Autodesk Inventor part; units mm, degrees
ref_plane "Work Plane1" through (0, 1.5, 0) normal (0, -1, 0) x (1, 0, 0)
ref_plane "YZ Plane" through (0, 0, 0) normal (1, 0, 0) x (0, 1, 0)
ref_plane "XZ Plane" through (0, 0, 0) normal (0, 1, 0) x (-1, 0, 0)
sketch "Sketch1" plane through (0, 0, 0) normal (0, 1, 0) x (-1, 0, 0)
  line L0 (0, 0) -> (29.5, 0)
  line L1 (29.5, 0) -> (29.5, -36.2)
  line L2 (29.5, -36.2) -> (0, -36.2)
  line L3 (0, -36.2) -> (0, 0)
  dimension "d0" = 29.5
  dimension "d1" = 36.2
extrude "Extrusion1" add sketch "Sketch1" along normal blind 5
sketch "Sketch2" plane through (0, 5, 0) normal (0, 1, 0) x (1, 0, 0)
  line L0 (-29.5, 0) -> (0, 0)
  line L1 (-14.75, 0) -> (-14.75, 17.5)
  arc A0 (-18.4298, 18.4481) -> (-11.0702, 18.4481) centre (-14.75, 17.5) ccw
  line L2 (-14.75, 17.5) -> (-14.75, 23.5)
  arc A1 (-11.0702, 18.4481) -> (-18.4298, 18.4481) centre (-14.75, 23.5) ccw
  circle A2 centre (-14.75, 23.5) radius 12.175
  circle A3 centre (-14.75, 23.5) radius 14.75
  dimension "d4" = 17.5
  dimension "d5" = 7.6
  dimension "d6" = 6
  dimension "d7" = 12.5
  dimension "d8" = 24.35
  dimension "d9" = 29.5
extrude "Extrusion2" add sketch "Sketch2" along normal blind 3.8 contours A2 | A3
sketch "Sketch4" plane through (-14.75, 8.8, -23.5) normal (0, 1, 0) x (1, 0, 0)
  circle A0 centre (0, 0) radius 12.25
  circle A1 centre (0, 0) radius 14.7438
  point P0 (14.75, -23.5)
  dimension "d12" = 24.5
extrude "Extrusion3" add sketch "Sketch4" along normal blind 6
sketch "Sketch5" plane through (-14.75, 8.8, -23.5) normal (0, 1, 0) x (1, 0, 0)
  arc A0 (-3.6798, -5.0519) -> (3.6798, -5.0519) centre (0, -6) ccw
  arc A1 (3.6798, -5.0519) -> (-3.6798, -5.0519) centre (0, 0) ccw
  point P0 (14.75, -23.5)
extrude "Extrusion4" cut sketch "Sketch5" against normal up to surface (8.8 mm away)
sketch "Sketch6" plane through (0, 0, 0) normal (0, -1, 0) x (1, 0, 0)
  arc A0 (-11.0702, -18.4481) -> (-18.4298, -18.4481) centre (-14.75, -17.5) ccw
  arc A1 (-18.4298, -18.4481) -> (-11.0702, -18.4481) centre (-14.75, -23.5) ccw
  line L0 (0, 0) -> (-29.5, 0)
  line L1 (-29.5, 0) -> (-29.5, -36.2)
  line L2 (-29.5, -36.2) -> (0, -36.2)
  line L3 (0, -36.2) -> (0, 0)
  line L4 (-14.75, 0) -> (-14.75, -36.2)
  line L5 (0, -36.2) -> (0, 0)
  line L6 (0, -18.1) -> (-29.5, -18.1)
  line L7 (-21.0275, -1.55) -> (-8.4725, -1.55)
  line L8 (-8.4725, -1.55) -> (-8.4725, -34.65)
  line L9 (-8.4725, -34.65) -> (-21.0275, -34.65)
  line L10 (-21.0275, -34.65) -> (-21.0275, -1.55)
  line L11 (-21.0275, -1.55) -> (-8.4725, -34.65) construction
  line L12 (-8.4725, -1.55) -> (-21.0275, -34.65) construction
  point P0 (-14.75, -18.1)
  dimension "d17" = 12.555
  dimension "d18" = 33.1
extrude "Extrusion5" cut sketch "Sketch6" against normal blind 6 contours A0 L6 L8 L9 L4 A1 | A0 L4 L7 L8 L6 | L4 L9 L10 L6 A0 A1 | A0 L6 L10 L7 L4
ref_plane "Work Plane1" through (0, 1.5, 0) normal (0, -1, 0) x (1, 0, 0)
sketch "Sketch7" plane through (0, 1.5, 0) normal (0, -1, 0) x (1, 0, 0)
  line L0 (-8.4725, -1.55) -> (-8.4725, -34.65)
  line L1 (-8.4725, -34.65) -> (-21.0275, -34.65)
  line L2 (-21.0275, -1.55) -> (-8.4725, -1.55)
  line L3 (-21.0275, -34.65) -> (-21.0275, -1.55)
  line L4 (-8.4725, -1.55) -> (-21.0275, -1.55)
  line L5 (-21.0275, -1.55) -> (-21.0275, -6.091)
  line L6 (-21.0275, -6.091) -> (-8.4725, -6.091)
  line L7 (-8.4725, -6.091) -> (-8.4725, -1.55)
  line L8 (-8.4725, -34.65) -> (-21.0201, -34.65)
  line L9 (-21.0201, -34.65) -> (-21.0201, -30.109)
  line L10 (-21.0201, -30.109) -> (-8.4725, -30.109)
  line L11 (-8.4725, -30.109) -> (-8.4725, -34.65)
  line L12 (-14.75, -1.55) -> (-14.7463, -34.65)
  line L13 (-14.75, -1.55) -> (-14.7498, -3.632)
  line L14 (-14.7463, -34.65) -> (-14.7465, -32.568)
  circle A0 centre (-14.7498, -3.632) radius 1
  circle A1 centre (-14.7465, -32.568) radius 1
  point P0 (0, 0)
  dimension "d22" = 4.541
  dimension "d23" = 12.555
  dimension "d24" = 4.541
  dimension "d25" = 12.5476
  dimension "d26" = 2.082
  dimension "d27" = 0
  dimension "d28" = 2.082
  dimension "d29" = 0
  dimension "d30" = 2
  dimension "d31" = 2
extrude "Extrusion6" add sketch "Sketch7" against normal up to surface (3.5 mm away) contours L0 L6 L12 A0 L2 | L12 A0 L6 L3 L2 | L0 L1 L12 A1 L10 | L12 A1 L1 L9 L10
properties part number "middle"
Work out the finished part from the listing and answer in its coordinate system (mm). A direction names the side the tool comes from. Give positions to 0.01 mm unless a question says otherwise; leave off trailing zeros. Loops run counter-clockwise (first coordinate to the right, second up) from the corner with the lowest first, then second, coordinate; pieces in that order, holes last. Notation, with made-up numbers: M 24,9 L 83,9 A26 ccw 83,23 Z; hole C 54.5,40 d10. An arc over 180 degrees is marked long. One line per item, written item: value. Start each with the question number.
1. Find section C-C (x = -17.5). State how many separate pieces and enclosed holes the cut face has, and give its area (3 significant figures).
2. Determine the mould class of faces 4 (the face through (-29.5, 2, -18)), 5 (the face through (-13, 14.8, -36)), 6 (the face through (-15, 1, -1.55)) for opening direction X: released by +X, released by -X, zero draft, split by the parting line, or undercut.
3. Find section B-B (y = 12.5). Give the vertices of the cut face in (x, z), and give its area (3 significant figures).
4. Find the intervals of material crossed by probe 1 along X at (y, z) = (6.95, -23.5); probe 2 along Z at (x, y) = (-14.75, 8.2); probe 3 along X at (y, z) = (12.1, -23.5), in increasing order.
5. Find section A-A (z = -8). Give the vertices of the cut face in (x, y), and give its area (3 significant figures).
6. Which of the six approach directions +Z, -Z, +X, -X, +Y, -Y give full straight-line access (tool end or side, diameter ignored) to faces 1 (the face through (-27, 5, -33)), 2 (the face through (-2, 5, -33)), 3 (the face through (-15.54, 3.226, -33.176))?
7. Each of these flat-tipped pins is pushed along its axis until it touches: P1, Ø6, axis at x = -14.75, z = -17.5, coming from the +Y side; P2, Ø3, axis at x = -4, z = -11, coming from the -Y side; P3, Ø5, axis at x = -8.5, z = -25, coming from the +Y side; P4, Ø6, axis at y = 12.5, z = -30.5, coming from the -X side. Where does it stop, or does it pass through?
Reported:
1. separate pieces: 3
1. enclosed holes: 0
1. area: 122 mm²
2. face 4: released by -X
2. face 5: zero draft
2. face 6: undercut
3. outline: C -14.75,-23.5 d29.49; hole C -14.75,-23.5 d24.5
3. area: 211 mm²
4. probe 1: x = -29.5 to -21, -8.5 to 0
4. probe 2: z = -38.25 to -29.75, -13.7 to -8.75
4. probe 3: x = -29.49 to -27, -2.5 to -0.01
5. outline: M -29.5,0 L -21.03,0 L -21.03,5 L -29.5,5 Z; M -8.47,0 L 0,0 L 0,5 L -8.47,5 Z
5. area: 84.7 mm²
6. face 1: -Z, -X, +Y
6. face 2: -Z, +X, +Y
6. face 3: -Y
7. P1: passes through
7. P2: stops at y = 0
7. P3: stops at y = 8.8
7. P4: stops at x = -28.94
